Drawing for the job (mm, zero at the part's lowest x, y, z). Give positions to 0.01 mm unless a question says otherwise; leave off trailing zeros. Order: outer loops, then holes, each group sorted by start corner. A loop starts at its lowest first (then second) coordinate and runs counter-clockwise, first axis right, second up. Notation, with made-up numbers: (72, -12) - (105, -12) arc R10 ccw to (105, -8) - close; hole circle Ø10 at (-6, 73.25). An arc over 180 degrees is marked (long way). Use a Markdown table: item, result. Add a question column.
(1) Wall check: line 1 (X direction, y = 0.5, z = 5.5); line 2 (X direction, y = 3.75, z = 29.5); line 3 (Y direction, x = 5, z = 47). Give the ranges that are in metal, low to high.
(2) Flat gauge pins, fed straight in: pin 1 (2 mm diameter, centred on y = 2, z = 26, fed in from +X); pin 2 (1.5 mm diameter, centred on y = 1.5, z = 13.5, fed in from +X) (1 decimal). Where does each tip first touch, or does it go through?
(3) Slice it at C-C (x = 1.25). Write the cut outline in (y, z).
(4) Slice it at B-B (y = 5). Write the cut outline in (x, z) (1 decimal).
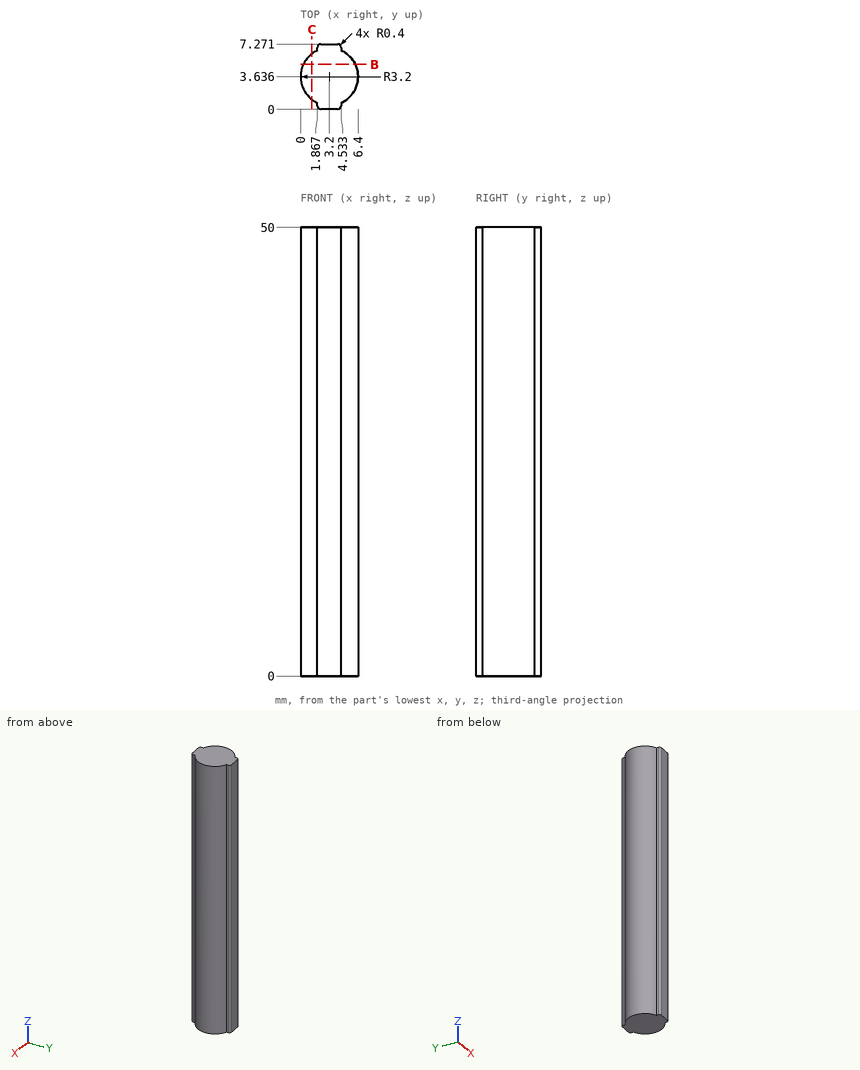
Solution:
| question | item | result |
|---|---|---|
| 1 | line 1 | 1.87 to 4.53 |
| 1 | line 2 | 0 to 6.4 |
| 1 | line 3 | 0.99 to 6.28 |
| 2 | pin 1 | x = 6.34 |
| 2 | pin 2 | x = 6.1 |
| 3 | outline | (1.1, 0) - (6.17, 0) - (6.17, 50) - (1.1, 50) - close |
| 4 | outline | (0.3, 0) - (6.1, 0) - (6.1, 50) - (0.3, 50) - close |
